The drawing under review shows one solid part. Ordinate dimensions are in mm from its lowest x, y, z. A direction names the side the tool comes from. Round coordinates to 2 decimals unless told otherwise and drop trailing zeros. Loops run counter-clockwise (first coordinate to the right, second up) from the corner with the lowest first, then second, coordinate; pieces in that order, holes last. Notation, with made-up numbers: (88.25, 3) -> (95.25, 3) arc R28 cw to (95.25, 27) -> close; hole circle Ø10 at (6, 65.25). An arc over 180 degrees is marked (long way). Use a Markdown table: item, result. Add a question column.
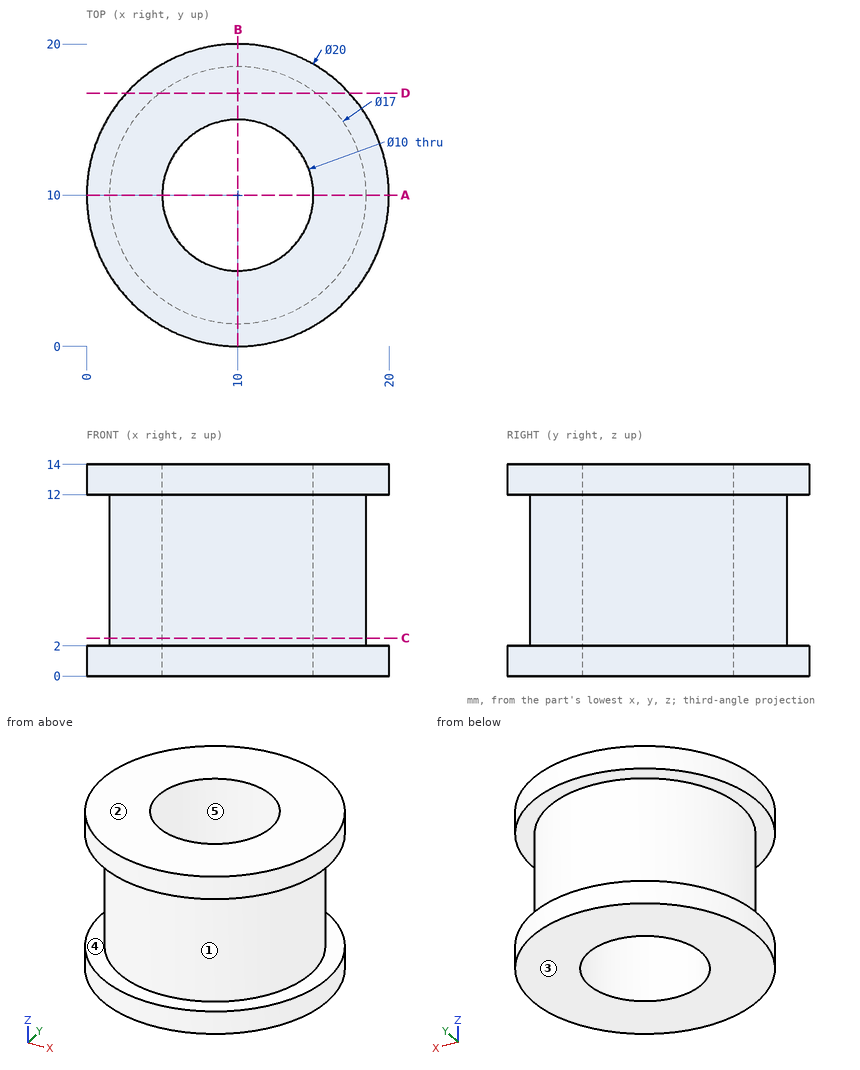
1. To check wall thickness, follow probe 1 along Z at (x, y) = (3.25, 17); probe 2 along Y at (x, z) = (10, 6.25); probe 3 along X at (y, z) = (11.25, 8). State the ranges of each line that lie inside material, in increasing order. Write a range as from..to.
2. Insertion check: P1, Ø4, axis at x = 12.5, z = 12.5, coming from the +Y side; P2, Ø2, axis at x = 13, z = 2.5, coming from the -Y side; P3, Ø1.5, axis at x = 15, z = 11.5, coming from the -Y side. Each pin has a flat end and moves straight along its axis. Give the tip position at first contact, or say it passes through.
3. For the marked faces 1 and 2, list the 3-axis set-ups (+Z, -Z, +X, -X, +Y, -Y) from which the entire face can be reached by the end or side of a thin tool; tool diameter is ignored.
4. Mouldability with a two-part tool opening along Z and no side actions: class the marked faces 3, 4 and 5 as +Z half, -Z half, draft (parallel to the pull), parting line (faces both ways), or undercut.
5. Consider section A-A on y = 10. State the section outline as (x, z) points.
6. Consider section D-D on y = 16.75. State the section outline as (x, z) points.
7. Consider section C-C on z = 2.5. State the section outline as (x, y) points.
Verdict:
| question | item | result |
|---|---|---|
| 1 | probe 1 | z = 0..2, 12..14 |
| 1 | probe 2 | y = 1.5..5, 15..18.5 |
| 1 | probe 3 | x = 1.59..5.16, 14.84..18.41 |
| 2 | P1 | stops at y = 19.99 |
| 2 | P2 | stops at y = 0.23 |
| 2 | P3 | stops at y = 1.04 |
| 3 | face 1 | none |
| 3 | face 2 | +Z, +X, -X, +Y, -Y |
| 4 | face 3 | -Z half |
| 4 | face 4 | undercut |
| 4 | face 5 | draft |
| 5 | outline | (0, 0) -> (5, 0) -> (5, 14) -> (0, 14) -> (0, 12) -> (1.5, 12) -> (1.5, 2) -> (0, 2) -> close; (15, 0) -> (20, 0) -> (20, 2) -> (18.5, 2) -> (18.5, 12) -> (20, 12) -> (20, 14) -> (15, 14) -> close |
| 6 | outline | (2.62, 0) -> (17.38, 0) -> (17.38, 2) -> (15.17, 2) -> (15.17, 12) -> (17.38, 12) -> (17.38, 14) -> (2.62, 14) -> (2.62, 12) -> (4.83, 12) -> (4.83, 2) -> (2.62, 2) -> close |
| 7 | outline | circle Ø17 at (10, 10); hole circle Ø10 at (10, 10) |
